from build123d import *

# Parameters (mm, degrees)
SKETCH1_W           = 103.6
SKETCH1_H           = 55.42
BOSS_EXTRUDE1_DEPTH = 1.5
SKETCH2_R           = 1
CUT_EXTRUDE1_DEPTH  = 1.5
BOSS_EXTRUDE2_DEPTH = 17
BOSS_EXTRUDE4_DEPTH = 10
CUT_EXTRUDE2_DEPTH  = 15


with BuildPart() as part:
    # Sketch1 → Boss-Extrude1 (new body)
    with BuildSketch(Plane.XY):
        with Locations((51.8, 27.71)):
            Rectangle(SKETCH1_W, SKETCH1_H)
    extrude(amount=BOSS_EXTRUDE1_DEPTH)

    # Sketch2 → Cut-Extrude1 (cut)
    with BuildSketch(Plane(origin=(0, 0, 0), x_dir=(-1, 0, 0), z_dir=(0, 0, -1))):
        with Locations((-90.42, 3.54)):
            Circle(SKETCH2_R)
        with Locations((-15.28, 3.54)):
            Circle(SKETCH2_R)
        with Locations((-97.91, 51.88)):
            Circle(SKETCH2_R)
        with Locations((-15.28, 51.88)):
            Circle(SKETCH2_R)
    extrude(amount=-CUT_EXTRUDE1_DEPTH, mode=Mode.SUBTRACT)

    # Sketch3 → Boss-Extrude2 (add)
    with BuildSketch(Plane.XY.offset(1.5)):
        Polygon((9.663353886, 41.72), (15.610061659, 41.72), (18.583415545, 46.87), (15.610061659, 52.02), (9.663353886, 52.02), (6.69, 46.87), align=None)
        Polygon((6.69, 8.67), (9.663353886, 13.82), (15.610061659, 13.82), (18.583415545, 8.67), (15.610061659, 3.52), (9.663353886, 3.52), align=None)
        Polygon((96.776831091, 46.87), (93.803477204, 41.72), (87.856769432, 41.72), (84.883415545, 46.87), (87.856769432, 52.02), (93.803477204, 52.02), align=None)
        Polygon((93.803477204, 13.82), (87.856769432, 13.82), (84.883415545, 8.67), (87.856769432, 3.52), (93.803477204, 3.52), (96.776831091, 8.67), align=None)
    extrude(amount=BOSS_EXTRUDE2_DEPTH)

    # Sketch4 → Boss-Extrude4 (add)
    with BuildSketch(Plane.XY.offset(1.5)):
        Polygon((20.199996299, 46.87), (17.267876695, 51.948580128), (16.418352036, 53.42), (14.289848496, 53.42), (8.855063509, 53.42), (5.073419246, 46.87), (8.855063509, 40.32), (16.418352036, 40.32), align=None)
        Polygon((18.583415545, 46.87), (16.05544113, 51.248580128), (15.610061659, 52.02), (14.289848496, 52.02), (9.663353886, 52.02), (6.69, 46.87), (9.663353886, 41.72), (15.610061659, 41.72), align=None, mode=Mode.SUBTRACT)
        Polygon((8.855063509, 2.12), (14.28020002, 2.12), (16.418352036, 2.12), (17.226260541, 3.519338579), (20.199996299, 8.67), (16.418352036, 15.22), (8.855063509, 15.22), (5.073419246, 8.67), align=None)
        Polygon((9.663353886, 3.52), (14.28020002, 3.52), (15.610061659, 3.52), (16.013824976, 4.219338579), (18.583415545, 8.67), (15.610061659, 13.82), (9.663353886, 13.82), (6.69, 8.67), align=None, mode=Mode.SUBTRACT)
        Polygon((83.266834792, 8.67), (87.048479055, 2.12), (89.42020002, 2.12), (91.41979998, 2.12), (94.611767581, 2.12), (98.393411844, 8.67), (94.611767581, 15.22), (87.048479055, 15.22), align=None)
        Polygon((84.883415545, 8.67), (87.856769432, 3.52), (89.42020002, 3.52), (91.41979998, 3.52), (93.803477204, 3.52), (96.776831091, 8.67), (93.803477204, 13.82), (87.856769432, 13.82), align=None, mode=Mode.SUBTRACT)
        Polygon((98.393411844, 46.87), (94.611767581, 53.42), (87.048479055, 53.42), (83.266834792, 46.87), (87.048479055, 40.32), (94.611767581, 40.32), align=None)
        Polygon((96.776831091, 46.87), (93.803477204, 52.02), (87.856769432, 52.02), (84.883415545, 46.87), (87.856769432, 41.72), (93.803477204, 41.72), align=None, mode=Mode.SUBTRACT)
    extrude(amount=BOSS_EXTRUDE4_DEPTH)

    # Sketch5 → Cut-Extrude2 (cut)
    with BuildSketch(Plane.XY.offset(18.5)):
        Polygon((14.801771282, 50.62), (10.471644263, 50.62), (8.306580754, 46.87), (10.471644263, 43.12), (14.801771282, 43.12), (16.966834792, 46.87), align=None)
        Polygon((88.665059808, 43.12), (92.995186827, 43.12), (95.160250337, 46.87), (92.995186827, 50.62), (88.665059808, 50.62), (86.499996299, 46.87), align=None)
        Polygon((88.665059808, 4.92), (92.995186827, 4.92), (95.160250337, 8.67), (92.995186827, 12.42), (88.665059808, 12.42), (86.499996299, 8.67), align=None)
        Polygon((14.801771282, 12.42), (10.471644263, 12.42), (8.306580754, 8.67), (10.471644263, 4.92), (14.801771282, 4.92), (16.966834792, 8.67), align=None)
    extrude(amount=-CUT_EXTRUDE2_DEPTH, mode=Mode.SUBTRACT)


solid = part.part
Check sheet for the modelled part. Datum: model origin and axes. Units: mm. A direction names the side the tool comes from. Give positions to 0.01 mm unless a question says otherwise; leave off trailing zeros. Loops run counter-clockwise (first coordinate to the right, second up) from the corner with the lowest first, then second, coordinate; pieces in that order, holes last. Notation, with made-up numbers: M 80.25,-31 L 111.25,-31 A13 ccw 111.25,-21 Z; hole C 2.5,84 d11. An arc over 180 degrees is marked long. Answer as a JSON object with one key per item and string values. Group by question number.
Q1. Go/stop test with flat-tipped pins: P1, Ø4, axis at x = 91, z = 4.5, coming from the -Y side; P2, Ø4, axis at x = 92, y = 47.5, coming from the +Z side; P3, Ø12, axis at x = 27, y = 28.5, coming from the +Z side. Record where each tip stops, or that it passes through.
Q2. Cross-section at A-A on z = 9.5. Give the number of separate pieces and of enclosed holes in the cut face, then the cut area to 3 significant figures.
Q3. Cross-section at C-C on y = 19.5. Record the cut outline in (x, z).
Q4. Material ranges on line 1 along Y through (x, z) = (15.28, 1.1); line 2 along Y through (x, z) = (90.42, 0.9); line 3 along X through (y, z) = (6, 11), recorded low to high. Write a range as [from, to].
Q5. Access from +Z, -Z, +X, -X, +Y, -Y to the whole of each face (thin tool, end or side, straight path). Record for faces 1 (the flat face through (91, 40.32, 6)), 2 (the flat face through (15.9, 10.52, 11.1)), 3 (the flat face through (15, 4, 1.5)).
Q6. Release check for a two-part mould opening along Y. For faces 4 (the flat face through (17.1, 5.8, 11.5)), 5 (the flat face through (91, 3.52, 15)), 6 (the flat face through (95.27, 49.48, 14.95)) record: released by +Y, released by -Y, zero draft, split by the parting line, or undercut.
Evaluation:
{
 "1": {"P1": "stops at y = 2.12", "P2": "stops at z = 3.5", "P3": "stops at z = 1.5"},
 "2": {"separate pieces": "4", "enclosed holes": "4", "area": "400 mm2"},
 "3": {"outline": "M 0,0 L 103.6,0 L 103.6,1.5 L 0,1.5 Z"},
 "4": {"line 1": "y = [0, 2.54], [4.54, 50.88], [52.88, 55.42]", "line 2": "y = [0, 2.54], [4.54, 55.42]", "line 3": "x = [6.61, 9.85], [15.43, 18.66], [84.81, 88.04], [93.62, 96.85]"},
 "5": {"face 1": "+Z, +X, -X", "face 2": "+Z", "face 3": "-Z"},
 "6": {"face 4": "undercut", "face 5": "released by -Y", "face 6": "released by +Y"}
}
